Source: CAD feature listing. Evaluate the final solid. Frame: model axes, mm. A direction names the side the tool comes from. Coordinates: 2 decimals unless noted, no trailing zeros. Loops run counter-clockwise (first coordinate to the right, second up) from the corner with the lowest first, then second, coordinate; pieces in that order, holes last.
Item 1: Pin query (flat end, axial travel): pin 1 Ø1 at (y, z) = (1.5, -1.5) entering from -X; pin 2 Ø5 at (x, z) = (0, 0) entering from +Y. Return the tip coordinate at first contact, or that it passes through.
Item 2: Line query: probe 1 along X at (y, z) = (1.9, -25.4) (3 decimals); probe 2 along Z at (x, y) = (-43, 1); probe 3 along X at (y, z) = (0.55, -28). Output: solid intervals per line, ascending.
Item 3: Pull-direction query (X, two-part tool) for faces 3 (the cylindrical face through (-1.93, 1.61, -2.52)), 4 (the flat face through (12.7, 2, 1)), 5 (the flat face through (-12.7, 2, 0)); classes: +X half, -X half, draft (parallel to the pull), parting line (faces both ways), or undercut.
Item 4: Section query C-C, the plane y = 2.55. State how many separate pieces and enclosed holes the cut face has, then the cut area to 3 significant figures.
Item 5: Section query B-B, the plane x = -30.5. Return the cut outline in (y, z) (3 decimals).
Item 6: Reachability of faces 1 (the cylindrical face through (-0.95, 1.61, 9.67)), 2 (the flat face through (-41, 2, -12.7)) from +Z, -Z, +X, -X, +Y, -Y: full face, straight path, thin tool, end or side. Return the list, or none.
Item 7: Section query D-D, the plane z = -25.4. Return the cut outline in (x, y) (3 decimals).
Item 8: Section query A-A, the plane z = 0. Return the cut outline in (x, y) (3 decimals), then the cut area to 3 significant figures.
```python
from build123d import *

# Parameters (mm, degrees)
BOSS_EXTRUDE1_DEPTH = 3.175
SKETCH2_R           = 3.175
CUT_EXTRUDE1_DEPTH  = 75.121121315
FILLET1_R           = 1.5875
FILLET2_R           = 6.35


with BuildPart() as part:
    # Sketch1 → Boss-Extrude1 (new body)
    with BuildSketch(Plane(origin=(0, 0, 0), x_dir=(1, 0, 0), z_dir=(0, 1, 0))):
        Polygon((-12.7, -38.1), (12.7, -38.1), (12.7, 38.1), (-12.7, 38.1), (-63.5, 38.1), (-63.5, 12.7), (-12.7, 12.7), (-12.7, -12.7), (-63.5, -12.7), (-63.5, -38.1), align=None)
    extrude(amount=BOSS_EXTRUDE1_DEPTH)

    # Sketch2 → Cut-Extrude1 (cut, through all)
    with BuildSketch(Plane(origin=(0, 3.175, 0), x_dir=(1, 0, 0), z_dir=(0, 1, 0))):
        with Locations(Location((0, 0, 0), (0, 0, 270))):
            Circle(SKETCH2_R)
        with Locations(Location((0, 12.7, 0), (0, 0, 270))):
            Circle(SKETCH2_R)
        with Locations(Location((0, 25.4, 0), (0, 0, 270))):
            Circle(SKETCH2_R)
        with Locations(Location((0, -25.4, 0), (0, 0, 90))):
            Circle(SKETCH2_R)
        with Locations(Location((0, -12.7, 0), (0, 0, 90))):
            Circle(SKETCH2_R)
        with Locations(Location((-50.8, 25.4, 0), (0, 0, 270))):
            Circle(SKETCH2_R)
        with Locations(Location((-38.1, 25.4, 0), (0, 0, 270))):
            Circle(SKETCH2_R)
        with Locations(Location((-25.4, 25.4, 0), (0, 0, 270))):
            Circle(SKETCH2_R)
        with Locations(Location((-25.4, -25.4, 0), (0, 0, 90))):
            Circle(SKETCH2_R)
        with Locations(Location((-38.1, -25.4, 0), (0, 0, 90))):
            Circle(SKETCH2_R)
        with Locations(Location((-50.8, -25.4, 0), (0, 0, 90))):
            Circle(SKETCH2_R)
    extrude(amount=-CUT_EXTRUDE1_DEPTH, mode=Mode.SUBTRACT)

    # Fillet1
    fillet1_edges = [part.edges().sort_by_distance(p)[0] for p in [
        (12.7, 1.5875, 38.1),
        (-63.5, 1.5875, 38.1),
        (-63.5, 1.5875, 12.7),
        (-63.5, 1.5875, -12.7),
        (-63.5, 1.5875, -38.1),
        (12.7, 1.5875, -38.1),
    ]]
    fillet(fillet1_edges, radius=FILLET1_R)

    # Fillet2
    fillet2_edges = [part.edges().sort_by_distance(p)[0] for p in [
        (-12.7, 1.5875, 12.7),
        (-12.7, 1.5875, -12.7),
    ]]
    fillet(fillet2_edges, radius=FILLET2_R)


solid = part.part
```
Verdict:
1. pin 1: stops at x = -12.7
1. pin 2: passes through
2. probe 1: x = -63.5 to -53.975, -47.625 to -41.275, -34.925 to -28.575, -22.225 to -3.175, 3.175 to 12.7
2. probe 2: z = -38.1 to -12.7, 12.7 to 38.1
2. probe 3: x = -63.5 to -52.62, -48.98 to -39.92, -36.28 to -27.22, -23.58 to -1.82, 1.82 to 12.7
3. face 3: undercut
3. face 4: +X half
3. face 5: -X half
4. separate pieces: 1
4. enclosed holes: 11
4. area: 4,180 mm2
5. outline: (0, -38.1) - (3.175, -38.1) - (3.175, -12.7) - (0, -12.7) - close; (0, 12.7) - (3.175, 12.7) - (3.175, 38.1) - (0, 38.1) - close
6. face 1: +Y, -Y
6. face 2: -X, +Y, -Y
7. outline: (-63.5, 0) - (-53.975, 0) - (-53.975, 3.175) - (-63.5, 3.175) - close; (-47.625, 0) - (-41.275, 0) - (-41.275, 3.175) - (-47.625, 3.175) - close; (-34.925, 0) - (-28.575, 0) - (-28.575, 3.175) - (-34.925, 3.175) - close; (-22.225, 0) - (-3.175, 0) - (-3.175, 3.175) - (-22.225, 3.175) - close; (3.175, 0) - (12.7, 0) - (12.7, 3.175) - (3.175, 3.175) - close
8. outline: (-12.7, 0) - (-3.175, 0) - (-3.175, 3.175) - (-12.7, 3.175) - close; (3.175, 0) - (12.7, 0) - (12.7, 3.175) - (3.175, 3.175) - close
8. area: 60.5 mm2
